Part model, mm, in its own coordinate system. Face numbers are marked on the shaded views. Give positions to 0.01 mm unless a question says otherwise; leave off trailing zeros. Write each loop counter-clockwise with the first axis right and the second up, starting at its lowest first coordinate (ties: lowest second). Pieces come first, ordered by that corner, then holes.
from build123d import *

# Parameters (mm, degrees)
F0_R        = 12.5
F1_DEPTH    = 20
F2_R        = 3.625
F3_DEPTH    = 19.5
F4_SIZE     = 1.5
F5_SIZE     = 0.5
F6_W        = 1
F6_H        = 1
F8_T4_ANGLE = 270
F8_T6_ANGLE = 90


# Not quite as in the source:
# - a fillet or chamfer that OpenCascade refuses, or shapes differently, is made with other operations: its cross-section is extruded or revolved along the edge and cut away or added


with BuildPart() as f1:
    # F0 (on Top) → F1 (new body)
    with BuildSketch(Plane.XY):
        Circle(F0_R)
    extrude(amount=F1_DEPTH)

    # F2 (on Top) → F3 (cut)
    with BuildSketch(Plane.XY):
        Circle(F2_R)
    extrude(amount=F3_DEPTH, mode=Mode.SUBTRACT)

    # F4
    f4_edges = [f1.edges().sort_by_distance(p)[0] for p in [
        (-12.5, 0, 20),
    ]]
    chamfer(f4_edges, length=F4_SIZE)

    # F5
    f5_edges = [f1.edges().sort_by_distance(p)[0] for p in [
        (-12.5, 0, 0),
        (-3.625, 0, 0),
    ]]
    chamfer(f5_edges, length=F5_SIZE)

    # F6 (on Right) → F7 (revolve, cut)
    with BuildSketch(Plane.YZ):
        Polygon((12.5177614391, 14.5), (12.5177614391, 15.5), (11.5177614391, 15.5), (11.5177614391, 14.5179004222), align=None)
        with Locations((12.0177614391, 11)):
            Rectangle(F6_W, F6_H)
    revolve(axis=Axis((0, 0, 0), (0, 0, -1)), mode=Mode.SUBTRACT)

    # F8: chamfer of 0.2 on 5 edges, made by hand

    # F8_s1 → F8_t2 (revolve, cut)
    with BuildSketch(Plane.XZ):
        Polygon((12.3, 15.5), (12.5, 15.7), (12.5, 15.5), align=None)
    revolve(axis=Axis((0, 0, 15.5), (0, 0, -1)), mode=Mode.SUBTRACT)

    # F8_s3 → F8_t4 (revolve, cut)
    with BuildSketch(Plane.XZ):
        Polygon((12.5, 14.3038659818), (12.303579511, 14.5038339469), (12.5, 14.5003179373), align=None)
    revolve(axis=Axis((0, 0, 14.5003179373), (0, 0, -1)), revolution_arc=F8_T4_ANGLE, mode=Mode.SUBTRACT)

    # F8_s5 → F8_t6 (revolve, cut)
    with BuildSketch(Plane.YZ):
        Polygon((12.5, 14.3038659818), (12.303579511, 14.5038339469), (12.5, 14.5003179373), align=None)
    revolve(axis=Axis((0, 0, 14.5003179373), (0, 0, -1)), revolution_arc=F8_T6_ANGLE, mode=Mode.SUBTRACT)

    # F8_s7 → F8_t8 (revolve, cut)
    with BuildSketch(Plane.XZ):
        Polygon((12.3, 11.5), (12.5, 11.7), (12.5, 11.5), align=None)
    revolve(axis=Axis((0, 0, 11.5), (0, 0, -1)), mode=Mode.SUBTRACT)

    # F8_s9 → F8_t10 (revolve, cut)
    with BuildSketch(Plane.XZ):
        Polygon((12.5, 10.3), (12.3, 10.5), (12.5, 10.5), align=None)
    revolve(axis=Axis((0, 0, 10.5), (0, 0, -1)), mode=Mode.SUBTRACT)


solid = f1.part
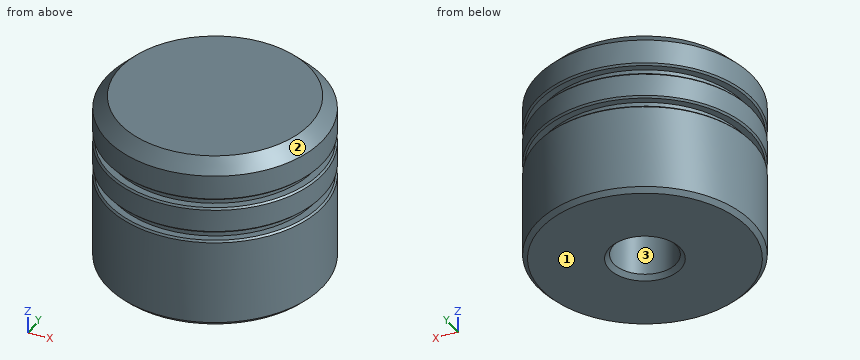
1) Drill centre lines: L1, parallel to Y at x = 0, z = 13.75 (3 decimals); L2, parallel to Z at x = 6.25, y = 9.75; L3, parallel to Z at x = 10, y = 6.75. Where is each one in solid material? Low to high.
Check result:
L1: y = -12.5 to -3.625, 3.625 to 12.5
L2: z = 0 to 10.5, 11.5 to 14.52, 15.5 to 19.42
L3: z = 0.06 to 10.5, 11.5 to 14.51, 15.5 to 18.94
2) Saw through at A-A (z = 5.25). Write the cut outline in (x, y) (3 decimals).
Check result:
outline: circle Ø25 at (0, 0); hole circle Ø7.25 at (0, 0)
3) Mould opens along X. For the marked faces 1, 2 and 3 say: +X half, -X half, draft (parallel to the pull), parting line (faces both ways), or undercut.
Check result:
face 1: draft
face 2: parting line
face 3: undercut
4) Flat gauge pins, fed straight in: P1, Ø5, axis at x = -8.5, z = 17.5, coming from the +Y side; P2, Ø4, axis at x = 6.5, z = 5.5, coming from the -Y side; P3, Ø3, axis at x = -9, z = 10, coming from the -Y side. Where does each tip first touch, or does it go through?
Check result:
P1: stops at y = 10.97
P2: stops at y = -11.66
P3: stops at y = -10
